Design review of the part built by this model. Coordinates are the model's own, in mm. A direction names the side the tool comes from. Round coordinates to 2 decimals unless told otherwise and drop trailing zeros. Write each loop counter-clockwise with the first axis right and the second up, starting at its lowest first coordinate (ties: lowest second). Pieces come first, ordered by that corner, then holes. Notation, with made-up numbers: M 40.25,55 L 46.25,55 A32 ccw 46.25,89 Z; hole C 64,-15.5 d9. An arc over 180 degrees is marked long. Use CSV: the item, a comma, the result in double quotes.
from build123d import *

# Parameters (mm, degrees)
BOX059_W                   = 15
BOX059_H                   = 6
BOX059_DEPTH               = 4
EXTRUDE027_DEPTH           = 5
EXTRUDE027_ROLL_ANGLE      = -90
EXTRUDE027_PLACEMENT_ANGLE = -90
CYLINDER053_R              = 1.6
CYLINDER053_DEPTH          = 10
CYLINDER052_R              = 1.6
CYLINDER052_DEPTH          = 10
SKETCH024_W                = 106.75
SKETCH024_H                = 41.75
SKETCH024_R                = 1.55
EXTRUDE024_DEPTH           = 8
EXTRUDE024_PLACEMENT_ANGLE = 270
BOX058_W                   = 6
BOX058_H                   = 17
BOX058_DEPTH               = 23
BOX056_W                   = 6
BOX056_H                   = 21
BOX056_DEPTH               = 64
TUBE003_R                  = 4
TUBE003_R_2                = 1.5
TUBE003_DEPTH              = 12


with BuildPart() as cube034:
    # Box059 → Box059 (new body)
    with BuildSketch(Plane(origin=(66.5, -0.9, 22.75), x_dir=(1, 0, 0), z_dir=(0, 0, 1))):
        with Locations((7.5, 3)):
            Rectangle(BOX059_W, BOX059_H)
    extrude(amount=BOX059_DEPTH)


with BuildPart() as extrude027:
    # Sketch028 → Extrude027 (new body)
    with BuildSketch(Plane.YZ):
        Polygon((10.25, 66.5), (10.25, 43.25), (12.9, 43.25), (12.9, 20.25), (16.15, 20.25), (16.15, 15.25), (24.15, 15.25), (24.15, 20.25), (27.4, 20.25), (27.4, 43.25), (30, 43.25), (30, 66.5), align=None)
    extrude(amount=EXTRUDE027_DEPTH)


with BuildPart() as extrude027_1:
    # Extrude027 roll: moved
    add(extrude027.part.rotate(Axis((0, 0, 0), (1, 0, 0)), EXTRUDE027_ROLL_ANGLE))


with BuildPart() as extrude027_2:
    # Extrude027 placement: moved
    add(extrude027_1.part.moved(Location((0, 4, 40.25))).rotate(Axis((0, 4, 40.25), (0, 0, 1)), EXTRUDE027_PLACEMENT_ANGLE))


with BuildPart() as cylinder053:
    # Cylinder053 → Cylinder053 (new body)
    with BuildSketch(Plane(origin=(114, 6.5, 46), x_dir=(0, 0, 1), z_dir=(-1, 0, 0))):
        Circle(CYLINDER053_R)
    extrude(amount=CYLINDER053_DEPTH)


with BuildPart() as m3cyl:
    # Cylinder052 → Cylinder052 (new body)
    with BuildSketch(Plane(origin=(114, 6.5, -6), x_dir=(0, 0, 1), z_dir=(-1, 0, 0))):
        Circle(CYLINDER052_R)
    extrude(amount=CYLINDER052_DEPTH)

    # Fusion038: union Cylinder053
    add(cylinder053.part)


with BuildPart() as bottom001:
    # Sketch024 → Extrude024 (new body)
    with BuildSketch(Plane.YZ):
        with Locations((53.375, 20.875)):
            Rectangle(SKETCH024_W, SKETCH024_H)
        with Locations((3, 3)):
            Circle(SKETCH024_R, mode=Mode.SUBTRACT)
        with Locations((3, 38.75)):
            Circle(SKETCH024_R, mode=Mode.SUBTRACT)
        with Locations((103.75, 38.75)):
            Circle(SKETCH024_R, mode=Mode.SUBTRACT)
        with Locations((103.75, 3)):
            Circle(SKETCH024_R, mode=Mode.SUBTRACT)
    extrude(amount=EXTRUDE024_DEPTH)


with BuildPart() as bottom001_1:
    # Extrude024 placement: moved
    add(bottom001.part.moved(Location((0, 4, 0))).rotate(Axis((0, 4, 0), (0, 0, 1)), EXTRUDE024_PLACEMENT_ANGLE))


with BuildPart() as basemount001:
    # Box058 → Box058 (new body)
    with BuildSketch(Plane(origin=(106.75, 0, 9.5), x_dir=(1, 0, 0), z_dir=(0, 0, 1))):
        with Locations((3, 8.5)):
            Rectangle(BOX058_W, BOX058_H)
    extrude(amount=BOX058_DEPTH)


with BuildPart() as obj1:
    # Box056 → Box056 (new body)
    with BuildSketch(Plane(origin=(106.75, -4, -12), x_dir=(1, 0, 0), z_dir=(0, 0, 1))):
        with Locations((3, 10.5)):
            Rectangle(BOX056_W, BOX056_H)
    extrude(amount=BOX056_DEPTH)

    # Cut038: cut baseMOunt001
    add(basemount001.part, mode=Mode.SUBTRACT)

    # Fusion037: union Bottom001
    add(bottom001_1.part)

    # Cut039: cut m3Cyl
    add(m3cyl.part, mode=Mode.SUBTRACT)

    # Cut040: cut Extrude027
    add(extrude027_2.part, mode=Mode.SUBTRACT)

    # Cut041: cut Cube034
    add(cube034.part, mode=Mode.SUBTRACT)


with BuildPart() as bottom002:
    # Tube003 → Tube003 (new body)
    with BuildSketch(Plane(origin=(71, 12, 18.5), x_dir=(0, 0, -1), z_dir=(0, -1, 0))):
        Circle(TUBE003_R)
        Circle(TUBE003_R_2, mode=Mode.SUBTRACT)
    extrude(amount=TUBE003_DEPTH)

    # Fusion039: union obj1
    add(obj1.part)


solid = bottom002.part
1) Add section A-A on y = 15.25. Write out the cut boundary in (x, z), then the cut area to 3 significant figures.
Answers:
outline,"M 106.75,-12 L 112.75,-12 L 112.75,9.5 L 106.75,9.5 Z; M 106.75,32.5 L 112.75,32.5 L 112.75,52 L 106.75,52 Z"
area,"246 mm²"
2) Machinability: for faces 1 (the face through (81.5, 2, 25)), 2 (the face through (56, -4, 20)), 3 (the face through (110, 9, 9.5)), 4 (the face through (110, 7, 52)), 5 (the face through (53, 0, 41.75)), which of the approach directions +Z, -Z, +X, -X, +Y, -Y give a long, thin tool a straight path to every point of the face, cutting with its end or side? Answer none if there is none.
Answers:
face 1,"+Y"
face 2,"+Z, -Z, +X, -X, -Y"
face 3,"+X, +Y"
face 4,"+Z, +X, -X, +Y, -Y"
face 5,"+Z, -X, +Y, -Y"
3) Add section B-B on x = 3. Write out the cut boundary in (y, z), then the cut area to 3 significant figures.
Answers:
outline,"M -4,0 L 4,0 L 4,1.45 L -4,1.45 Z; M -4,4.55 L 4,4.55 L 4,37.2 L -4,37.2 Z; M -4,40.3 L 4,40.3 L 4,41.75 L -4,41.75 Z"
area,"284 mm²"
4) Wall thickness on line 1 along Z through (x, y) = (3, -2.25); line 2 along Y through (x, z) = (110.8, 46); line 3 along X through (y, z) = (0.25, 18.5): over which ranges is each line inside the solid? List them lowest first. Write a range as [from, to].
Answers:
line 1,"[0, 1.45], [4.55, 37.2], [40.3, 41.75]"
line 2,"[-4, 4.9], [8.1, 17]"
line 3,"[0, 15.25], [66.5, 106.75]"
5) For pin 1 Ø2.5 at (y, z) = (0.5, 25.5) entering from +X; pin 2 Ø2 at (y, z) = (4, 13) entering from +X; pin 3 Ø4 at (x, y) = (37, 2.5) entering from -Z; pin 4 Ø1 at (x, z) = (23.5, 13.5) entering from +Y, all flat-tipped, find the tip position at first contact; note any pin that passes through.
Answers:
pin 1,"x = 112.75"
pin 2,"x = 106.75"
pin 3,"z = 0"
pin 4,"y = -1"
6) Add section D-D on y = 1.5. Give the number of separate pieces and of enclosed holes in the cut face, then the cut area to 3 significant figures.
Answers:
separate pieces,"1"
enclosed holes,"5"
area,"3,780 mm²"
7) Add section C-C on z = 38.75. Write out the cut boundary in (x, y), then the cut area to 3 significant figures.
Answers:
outline,"M 0,-4 L 1.45,-4 L 1.45,4 L 0,4 Z; M 4.55,-4 L 102.2,-4 L 102.2,4 L 4.55,4 Z; M 105.3,-4 L 112.75,-4 L 112.75,17 L 106.75,17 L 106.75,4 L 105.3,4 Z"
area,"930 mm²"
8) The part is to be moulded in two halves that separate along X. For faces 6 (the face through (109.79, 4.94, 45.65)), 7 (the face through (32, 2, 27.35)), 8 (the face through (112.75, -1, 20)), 9 (the face through (67.095, 8.056, 19.367)), say which applies: released by +X, released by -X, zero draft, split by the parting line, or undercut.
Answers:
face 6,"zero draft"
face 7,"undercut"
face 8,"released by +X"
face 9,"split by the parting line"
